Job drawing, mm, ordinate dimensions from the low corner. One solid piece. A direction names the side the tool comes from. Give positions to 0.01 mm unless a question says otherwise; leave off trailing zeros. Loops run counter-clockwise (first coordinate to the right, second up) from the corner with the lowest first, then second, coordinate; pieces in that order, holes last. Notation, with made-up numbers: M 37.25,28.5 L 43.25,28.5 A25 ccw 43.25,64.5 Z; hole C 33,-22.75 d1. An arc over 180 degrees is marked long. Put each result on its own line as item: value.
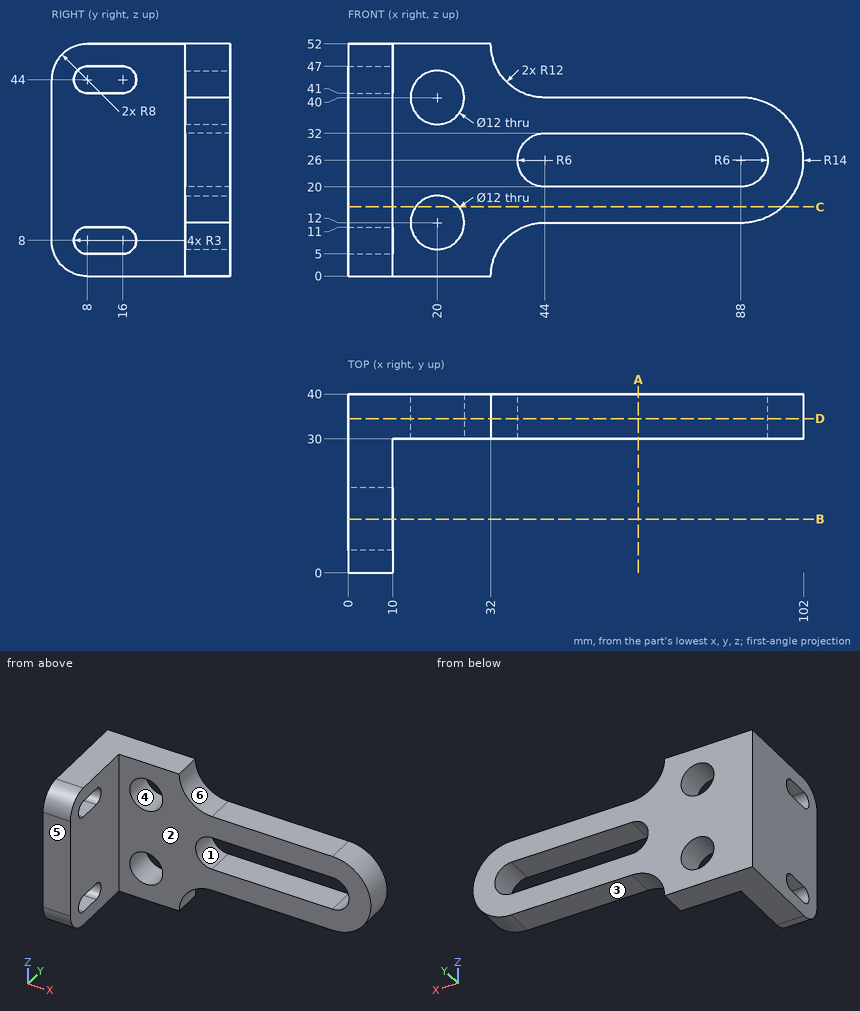
Q1. Slice it at C-C (z = 15.5). List the corners of the cut face in (x, y).
Here are the results:
outline: M 0,0 L 10,0 L 10,30 L 15.13,30 L 15.13,40 L 0,40 Z; M 24.87,30 L 97.26,30 L 97.26,40 L 24.87,40 Z
Q2. Slice it at B-B (y = 12). List the corners of the cut face in (x, z), and give its area (3 significant figures).
Here are the results:
outline: M 0,0 L 10,0 L 10,5 L 0,5 Z; M 0,11 L 10,11 L 10,41 L 0,41 Z; M 0,47 L 10,47 L 10,52 L 0,52 Z
area: 400 mm²
Q3. Slice it at A-A (x = 65). List the corners of the cut face in (y, z), and give its area (3 significant figures).
Here are the results:
outline: M 30,12 L 40,12 L 40,20 L 30,20 Z; M 30,32 L 40,32 L 40,40 L 30,40 Z
area: 160 mm²
Q4. Drop flat-ended pins along their axis: pin 1 Ø24 at (y, z) = (20, 17.5) entering from +X (3 decimals); pin 2 Ø8 at (x, y) = (74.5, 34) entering from -Z; pin 3 Ø8 at (x, y) = (85.5, 34) entering from +Z; pin 4 Ø10 at (x, z) = (43.5, 25.5) entering from -Y. Give the stop position or say it passes through.
Here are the results:
pin 1: x = 101.875
pin 2: z = 12
pin 3: z = 40
pin 4: through
Q5. Probe line 1 (Z direction, x = 20, y = 37.75); line 2 (Z direction, x = 46, y = 38); line 3 (Y direction, x = 60, z = 18). List the from-to ranges inside material, lowest first. Write a range as from..to.
Here are the results:
line 1: 0..6, 18..34, 46..52
line 2: 12..20, 32..40
line 3: 30..40
Q6. Tool access for the marked faces 1, 2 and 3: list every direction of +Z, -Z, +X, -X, +Y, -Y with a clear straight run to the whole face (end or side of a thin tool).
Here are the results:
face 1: +Y, -Y
face 2: +Z, -Z, +X, -Y
face 3: -Z, +X, +Y, -Y
Q7. Mould opens along Z. For the marked faces 4, 5 and 6 say: pulls with the +Z half, pulls with the -Z half, needs draft (parallel to the pull), parting line crosses it, or undercut.
Here are the results:
face 4: undercut
face 5: needs draft
face 6: pulls with the +Z half
Q8. Slice it at D-D (y = 34.5). State how many separate pieces and enclosed holes the cut face has, and give its area (3 significant figures).
Here are the results:
separate pieces: 1
enclosed holes: 3
area: 2,730 mm²
